```python
from build123d import *

# Parameters (mm, degrees)
SKETCH1_W           = 20
SKETCH1_H           = 40
BOSS_EXTRUDE1_DEPTH = 3
SKETCH2_R           = 4.1
CUT_EXTRUDE1_DEPTH  = 3
SKETCH3_W           = 12
SKETCH3_H           = 3
BOSS_EXTRUDE2_DEPTH = 40


with BuildPart() as part:
    # Sketch1 → Boss-Extrude1 (new body)
    with BuildSketch(Plane.XY):
        with Locations((0, 20)):
            Rectangle(SKETCH1_W, SKETCH1_H)
    extrude(amount=-BOSS_EXTRUDE1_DEPTH)

    # Sketch2 → Cut-Extrude1 (cut)
    with BuildSketch(Plane.XY):
        with Locations((0, 34)):
            Circle(SKETCH2_R)
    extrude(amount=-CUT_EXTRUDE1_DEPTH, mode=Mode.SUBTRACT)

    # Sketch3 → Boss-Extrude2 (add)
    with BuildSketch(Plane(origin=(0, 40, 0), x_dir=(1, 0, 0), z_dir=(0, 1, 0))):
        with Locations((0, 1.5)):
            Rectangle(SKETCH3_W, SKETCH3_H)
    extrude(amount=BOSS_EXTRUDE2_DEPTH)


solid = part.part
```
Here's how the part is built. I have some questions about the finished solid (model axes, mm). A direction names the side the tool comes from. Round coordinates to 2 decimals unless told otherwise and drop trailing zeros. Write each loop counter-clockwise with the first axis right and the second up, starting at its lowest first coordinate (ties: lowest second). Pieces come first, ordered by that corner, then holes. Notation, with made-up numbers: M 2.25,55.5 L 48.25,55.5 A27 cw 48.25,92.5 Z; hole C 41.25,87 d2. An arc over 180 degrees is marked long. Answer as CSV lines item,"result". Start each with the question number.
1. Suppose I cut it at D-D on y = 74. Write out the boundary of the cut face in (x, z), then the cut area to 3 significant figures.
2. I'm going to push flat-ended pins straight in: pin 1 Ø1.5 at (x, z) = (-7.5, -2) entering from +Y; pin 2 Ø1.5 at (y, z) = (59.5, -1) entering from -X. Where does each tip first touch, or does it pass through?
3. Suppose I cut it at B-B on x = 0. Write out the boundary of the cut face in (y, z).
4. Thinking about a two-plate mould opening in X: for faces 1 (the flat face through (-10, 20, -1)), 2 (the cylindrical face through (-3.022, 36.771, -1.479)), 3 (the flat face through (4, 32, 0)), which applies, released by +X, released by -X, zero draft, split by the parting line, or undercut?
5. I need wall thicknesses on probe 1 along Y at (x, z) = (0, -0.8); probe 2 along X at (y, z) = (66.5, -1.35); probe 3 along Y at (x, z) = (1, -0.8). Which ranges of each line are inside material? Lowest first, please.
6. On a 3-axis mill with a long thin cutter (end or side, diameter ignored), from which of +Z, -Z, +X, -X, +Y, -Y can I reach the whole of each face in a straight line? I mean faces 4 (the flat face through (0, 80, -2)), 5 (the flat face through (-6, 60, -1)), 6 (the flat face through (8, 40, -1)). Say none if no direction works.
7. Suppose I cut it at A-A on y = 34. Write out the boundary of the cut face in (x, z).
8. Suppose I cut it at C-C on z = -2.3. Write out the boundary of the cut face in (x, y).
Check result:
1,outline,"M -6,-3 L 6,-3 L 6,0 L -6,0 Z"
1,area,"36.0 mm2"
2,pin 1,"stops at y = 40"
2,pin 2,"stops at x = -6"
3,outline,"M 0,-3 L 29.9,-3 L 29.9,0 L 0,0 Z; M 38.1,-3 L 80,-3 L 80,0 L 38.1,0 Z"
4,face 1,"released by -X"
4,face 2,"undercut"
4,face 3,"zero draft"
5,probe 1,"y = 0 to 29.9, 38.1 to 80"
5,probe 2,"x = -6 to 6"
5,probe 3,"y = 0 to 30.02, 37.98 to 80"
6,face 4,"+Z, -Z, +X, -X, +Y"
6,face 5,"+Z, -Z, -X, +Y"
6,face 6,"+Z, -Z, +X, +Y"
7,outline,"M -10,-3 L -4.1,-3 L -4.1,0 L -10,0 Z; M 4.1,-3 L 10,-3 L 10,0 L 4.1,0 Z"
8,outline,"M -10,0 L 10,0 L 10,40 L 6,40 L 6,80 L -6,80 L -6,40 L -10,40 Z; hole C 0,34 d8.2"
